from build123d import *

# Parameters (mm, degrees)
SKETCH1_W           = 59.5
SKETCH1_H           = 80
SKETCH1_R           = 2.1
SKETCH1_R_2         = 2.6
BOSS_EXTRUDE1_DEPTH = 3
SKETCH2_R           = 2.5
CUT_EXTRUDE1_DEPTH  = 10


with BuildPart() as part:
    # Sketch1 → Boss-Extrude1 (new body)
    with BuildSketch(Plane(origin=(0, 0, 0), x_dir=(1, 0, 0), z_dir=(0, 1, 0))):
        Rectangle(SKETCH1_W, SKETCH1_H)
        with Locations(Location((24.5, 30, 0), (0, 0, 90))):
            Circle(SKETCH1_R, mode=Mode.SUBTRACT)
        with Locations(Location((-24.5, 30, 0), (0, 0, 270))):
            Circle(SKETCH1_R, mode=Mode.SUBTRACT)
        with Locations(Location((-24.5, 0, 0), (0, 0, 90))):
            Circle(SKETCH1_R, mode=Mode.SUBTRACT)
        with Locations(Location((24.5, 0, 0), (0, 0, 270))):
            Circle(SKETCH1_R, mode=Mode.SUBTRACT)
        with Locations(Location((9.75, -13, 0), (0, 0, 270))):
            Circle(SKETCH1_R_2, mode=Mode.SUBTRACT)
        with Locations(Location((-10.182503526, -13, 0), (0, 0, 270))):
            Circle(SKETCH1_R_2, mode=Mode.SUBTRACT)
    extrude(amount=BOSS_EXTRUDE1_DEPTH)

    # Sketch2 → Cut-Extrude1 (cut)
    with BuildSketch(Plane.XZ):
        with Locations(Location((-0.216251763, 30, 0), (0, 0, 270))):
            Circle(SKETCH2_R)
    extrude(amount=-CUT_EXTRUDE1_DEPTH, mode=Mode.SUBTRACT)


solid = part.part
The listing builds one solid part. Answer for the finished solid, in the listing's coordinates (mm). Give positions to 0.01 mm unless a question says otherwise; leave off trailing zeros. Loops run counter-clockwise (first coordinate to the right, second up) from the corner with the lowest first, then second, coordinate; pieces in that order, holes last. Notation, with made-up numbers: (77.5, 17) - (130.5, 17) arc R19 ccw to (130.5, 38) - close; hole circle Ø6 at (24, -16). An arc over 180 degrees is marked (long way). Answer as a JSON object with one key per item and string values.
1. Find the intervals of material crossed by L1, parallel to X at y = 2.2, z = -30; L2, parallel to X at y = 1.35, z = 13; L3, parallel to Z at x = 0, y = 1.55, in increasing order. Write a range as [from, to].
Determined:
{"L1": "[-29.75, -26.6], [-22.4, 22.4], [26.6, 29.75]", "L2": "[-29.75, -12.78], [-7.58, 7.15], [12.35, 29.75]", "L3": "[-40, 27.51], [32.49, 40]"}
2. A cutting plane is placed at D-D (z = -30). Write down the section's boundary in (x, y), then the cut area to 3 significant figures.
Determined:
{"outline": "(-29.75, 0) - (-26.6, 0) - (-26.6, 3) - (-29.75, 3) - close; (-22.4, 0) - (22.4, 0) - (22.4, 3) - (-22.4, 3) - close; (26.6, 0) - (29.75, 0) - (29.75, 3) - (26.6, 3) - close", "area": "153 mm²"}
3. A flat-ended cylindrical pin translates along its axis: pin 1 Ø3 at (x, z) = (-0.22, 30) entering from +Y. Find the tip coordinate at first contact, or state that the pin passes through.
Determined:
{"pin 1": "through"}
4. A cutting plane is placed at A-A (x = -24.5). Write down the section's boundary in (y, z).
Determined:
{"outline": "(0, -40) - (3, -40) - (3, -32.1) - (0, -32.1) - close; (0, -27.9) - (3, -27.9) - (3, -2.1) - (0, -2.1) - close; (0, 2.1) - (3, 2.1) - (3, 40) - (0, 40) - close"}
5. A cutting plane is placed at B-B (z = 30). Write down the section's boundary in (x, y).
Determined:
{"outline": "(-29.75, 0) - (-2.72, 0) - (-2.72, 3) - (-29.75, 3) - close; (2.28, 0) - (29.75, 0) - (29.75, 3) - (2.28, 3) - close"}
6. A cutting plane is placed at C-C (x = 9.75). Write down the section's boundary in (y, z).
Determined:
{"outline": "(0, -40) - (3, -40) - (3, 10.4) - (0, 10.4) - close; (0, 15.6) - (3, 15.6) - (3, 40) - (0, 40) - close"}
7. For a pull along X with two mould halves and no side action, classify faces 1 (the flat face through (-29.75, 1, 1)), 2 (the cylindrical face through (-0.106, 1.479, 32.498)), 3 (the flat face through (0, 1, -40)) as pulls with the +X half, pulls with the -X half, needs draft (parallel to the pull), parting line crosses it, or undercut.
Determined:
{"face 1": "pulls with the -X half", "face 2": "undercut", "face 3": "needs draft"}
